Here's how the part is built. I have some questions about the finished solid (model axes, mm). Give positions to 0.01 mm unless a question says otherwise; leave off trailing zeros. Loops run counter-clockwise (first coordinate to the right, second up) from the corner with the lowest first, then second, coordinate; pieces in that order, holes last. Notation, with made-up numbers: (-35, 72.25) - (-13, 72.25) arc R8 ccw to (-13, 86.25) - close; hole circle Ø9 at (18.25, 39.5). An arc over 180 degrees is marked (long way). Return JSON: item names as keys, results as strings. Group by question number.
(1) If we section it at C-C (z = 1.15): Please give me the cut outline in (x, y), then the cut area to 3 significant figures.
(2) For P1, Ø4.5, axis at x = -3, y = -28, coming from the +Z side; P2, Ø2, axis at x = 0, y = 0, coming from the +Z side, each with a flat end and sliding along its axis, tell me the tip position at first contact or that it passes through.
(3) If we mould it in two halves opening along X, with no side actions, what happens to faces 1 (the flat face through (-2, -33, 1)), 2 (the cylindrical face through (4.4, 19.43, 1.01)), 3 (the cylindrical face through (-2.11, -16.61, 0.99))? For each: released by +X, released by -X, zero draft, split by the parting line, or undercut.
(4) If we section it at B-B (x = -3): Please give me the cut outline in (y, z), then the cut area to 3 significant figures.
(5) I need wall thicknesses on probe 1 along Y at (x, z) = (0, 0.8); probe 2 along Y at (x, z) = (-3, 1.1); probe 3 along Y at (x, z) = (3.25, 0.6). Which ranges of each line are inside material? Lowest first, please. Write a range as [from, to].
(6) If we section it at A-A (y = 0): Please give me the cut outline in (x, z).
```python
from build123d import *

# Parameters (mm, degrees)
SKETCH_W  = 13
SKETCH_H  = 53
SKETCH_R  = 1.65
PAD_DEPTH = 2
FILLET_R  = 2


with BuildPart() as part:
    # Sketch → Pad (new body)
    with BuildSketch(Plane.XY):
        with Locations((-1.5, -6.5)):
            Rectangle(SKETCH_W, SKETCH_H)
        Circle(SKETCH_R, mode=Mode.SUBTRACT)
        with Locations((0, 10)):
            Circle(SKETCH_R, mode=Mode.SUBTRACT)
        with Locations((-3, -28)):
            Circle(SKETCH_R, mode=Mode.SUBTRACT)
        with Locations((-3, -18)):
            Circle(SKETCH_R, mode=Mode.SUBTRACT)
    extrude(amount=PAD_DEPTH)

    # Fillet
    fillet_edges = [part.edges().sort_by_distance(p)[0] for p in [
        (5, -33, 1),
        (-8, -33, 1),
        (5, 20, 1),
        (-8, 20, 1),
    ]]
    fillet(fillet_edges, radius=FILLET_R)


solid = part.part
```
Values:
{
 "1": {"outline": "(-8, -31) arc R2 ccw to (-6, -33) - (3, -33) arc R2 ccw to (5, -31) - (5, 18) arc R2 ccw to (3, 20) - (-6, 20) arc R2 ccw to (-8, 18) - close; hole circle Ø3.3 at (-3, -28); hole circle Ø3.3 at (-3, -18); hole circle Ø3.3 at (0, 0); hole circle Ø3.3 at (0, 10)", "area": "651 mm2"},
 "2": {"P1": "z = 2", "P2": "through"},
 "3": {"face 1": "zero draft", "face 2": "released by +X", "face 3": "undercut"},
 "4": {"outline": "(-33, 0) - (-29.65, 0) - (-29.65, 2) - (-33, 2) - close; (-26.35, 0) - (-19.65, 0) - (-19.65, 2) - (-26.35, 2) - close; (-16.35, 0) - (20, 0) - (20, 2) - (-16.35, 2) - close", "area": "92.8 mm2"},
 "5": {"probe 1": "[-33, -1.65], [1.65, 8.35], [11.65, 20]", "probe 2": "[-33, -29.65], [-26.35, -19.65], [-16.35, 20]", "probe 3": "[-32.98, 19.98]"},
 "6": {"outline": "(-8, 0) - (-1.65, 0) - (-1.65, 2) - (-8, 2) - close; (1.65, 0) - (5, 0) - (5, 2) - (1.65, 2) - close"}
}
